Geometry: final body of the model. Coordinates: model frame, mm. Coordinates: 2 decimals unless noted, no trailing zeros. Loops run counter-clockwise (first coordinate to the right, second up) from the corner with the lowest first, then second, coordinate; pieces in that order, holes last. Notation, with made-up numbers: (-9.5, 8) - (30.5, 8) arc R24 ccw to (30.5, 42) - close; hole circle Ø10 at (82, 30). An arc over 180 degrees is marked (long way). Put each result on its own line as item: value. Start each with the question number.
1) Section C-C on y = 0.45. Count the separate pieces of the cut face and the enclosed holes in it, and give its area (3 significant figures).
2) Material intervals for line 1 along X through (y, z) = (0.9, -11); line 2 along Z through (x, y) = (4.5, 0.4), sorted ascending. Write a range as from..to.
3) Draft query along X for faces 1 (the flat face through (-2.65, 1, -6)), 2 (the flat face through (6, 0, -9)), 3 (the flat face through (0, 1, -8.84)). Return one class per face: +X half, -X half, draft (parallel to the pull), parting line (faces both ways), or undercut.
4) Section A-A on x = -0.75. Output: boundary loops of the cut face in (y, z), and give its area (3 significant figures).
5) Section B-B on z = -14.25. Output: boundary loops of the cut face in (x, y).
```python
from build123d import *

# Parameters (mm, degrees)
SKETCH1_W           = 19.46
SKETCH1_H           = 19.46
SKETCH1_W_2         = 5.3
SKETCH1_H_2         = 5.3
BOSS_EXTRUDE1_DEPTH = 2.7


with BuildPart() as part:
    # Sketch1 → Boss-Extrude1 (new body)
    with BuildSketch(Plane(origin=(0, 0, 0), x_dir=(1, 0, 0), z_dir=(0, 1, 0))):
        with Locations((6.19, 6.19)):
            Rectangle(SKETCH1_W, SKETCH1_H)
        with Locations((6.19, 0)):
            Rectangle(SKETCH1_W_2, SKETCH1_H_2, mode=Mode.SUBTRACT)
        Rectangle(SKETCH1_W_2, SKETCH1_H_2, mode=Mode.SUBTRACT)
        with Locations((12.38, 0)):
            Rectangle(SKETCH1_W_2, SKETCH1_H_2, mode=Mode.SUBTRACT)
        with Locations((6.19, 6.19)):
            Rectangle(SKETCH1_W_2, SKETCH1_H_2, mode=Mode.SUBTRACT)
        with Locations((12.38, 6.19)):
            Rectangle(SKETCH1_W_2, SKETCH1_H_2, mode=Mode.SUBTRACT)
        with Locations((6.19, 12.38)):
            Rectangle(SKETCH1_W_2, SKETCH1_H_2, mode=Mode.SUBTRACT)
        with Locations((12.38, 12.38)):
            Rectangle(SKETCH1_W_2, SKETCH1_H_2, mode=Mode.SUBTRACT)
        with Locations((0, 6.19)):
            Rectangle(SKETCH1_W_2, SKETCH1_H_2, mode=Mode.SUBTRACT)
        with Locations((0, 12.38)):
            Rectangle(SKETCH1_W_2, SKETCH1_H_2, mode=Mode.SUBTRACT)
    extrude(amount=BOSS_EXTRUDE1_DEPTH)


solid = part.part
```
Answer block:
1. separate pieces: 1
1. enclosed holes: 9
1. area: 126 mm²
2. line 1: x = -3.54..-2.65, 2.65..3.54, 8.84..9.73, 15.03..15.92
2. line 2: z = -15.92..-15.03, -9.73..-8.84, -3.54..-2.65, 2.65..3.54
3. face 1: undercut
3. face 2: draft
3. face 3: undercut
4. outline: (0, -15.92) - (2.7, -15.92) - (2.7, -15.03) - (0, -15.03) - close; (0, -9.73) - (2.7, -9.73) - (2.7, -8.84) - (0, -8.84) - close; (0, -3.54) - (2.7, -3.54) - (2.7, -2.65) - (0, -2.65) - close; (0, 2.65) - (2.7, 2.65) - (2.7, 3.54) - (0, 3.54) - close
4. area: 9.61 mm²
5. outline: (-3.54, 0) - (-2.65, 0) - (-2.65, 2.7) - (-3.54, 2.7) - close; (2.65, 0) - (3.54, 0) - (3.54, 2.7) - (2.65, 2.7) - close; (8.84, 0) - (9.73, 0) - (9.73, 2.7) - (8.84, 2.7) - close; (15.03, 0) - (15.92, 0) - (15.92, 2.7) - (15.03, 2.7) - close
